from build123d import *

# Parameters (mm, degrees)
SKETCH1_R           = 6
BOSS_EXTRUDE2_DEPTH = 5
SKETCH2_W           = 36
SKETCH2_H           = 12
BOSS_EXTRUDE3_DEPTH = 48
CUT_EXTRUDE1_DEPTH  = 48
SKETCH4_R           = 7.2
CUT_EXTRUDE2_DEPTH  = 48
SKETCH5_R           = 7.2
CUT_EXTRUDE3_DEPTH  = 48


with BuildPart() as part:
    # Sketch1 → Boss-Extrude2 (new body, symmetric)
    with BuildSketch(Plane.XY):
        with BuildLine():
            Line((-48.497409326, 0), (47.502590674, 0))
            Line((47.502590674, 0), (11.523405954, 35.97918472))
            ThreePointArc((11.523405954, 35.97918472), (-0.497409326, 40.95836944), (-12.518224607, 35.97918472))
            Line((-12.518224607, 35.97918472), (-48.497409326, 0))
        make_face()
        with Locations((0, 15)):
            Circle(SKETCH1_R, mode=Mode.SUBTRACT)
    extrude(amount=BOSS_EXTRUDE2_DEPTH, both=True)

    # Sketch2 → Boss-Extrude3 (add, symmetric)
    with BuildSketch(Plane(origin=(0, 0, 0), x_dir=(0, 0, -1), z_dir=(1, 0, 0))):
        with Locations((-13, -6)):
            Rectangle(SKETCH2_W, SKETCH2_H)
    extrude(amount=BOSS_EXTRUDE3_DEPTH, both=True)

    # Sketch3 → Cut-Extrude1 (cut, symmetric)
    with BuildSketch(Plane(origin=(0, 0, 0), x_dir=(1, 0, 0), z_dir=(0, 1, 0))):
        with BuildLine():
            Line((-7, -23), (-7, -31))
            Line((-7, -31), (7, -31))
            Line((7, -31), (7, -23))
            ThreePointArc((7, -23), (4.949747468, -18.050252532), (0, -16))
            ThreePointArc((0, -16), (-4.949747468, -18.050252532), (-7, -23))
        make_face()
    extrude(amount=CUT_EXTRUDE1_DEPTH, both=True, mode=Mode.SUBTRACT)

    # Sketch4 → Cut-Extrude2 (cut, symmetric)
    with BuildSketch(Plane(origin=(0, 0, 0), x_dir=(1, 0, 0), z_dir=(0, 1, 0))):
        with Locations((-36, -18)):
            Circle(SKETCH4_R)
    extrude(amount=CUT_EXTRUDE2_DEPTH, both=True, mode=Mode.SUBTRACT)

    # Sketch5 → Cut-Extrude3 (cut, symmetric)
    with BuildSketch(Plane(origin=(0, 0, 0), x_dir=(1, 0, 0), z_dir=(0, 1, 0))):
        with Locations((36, -18)):
            Circle(SKETCH5_R)
    extrude(amount=CUT_EXTRUDE3_DEPTH, both=True, mode=Mode.SUBTRACT)


solid = part.part
Design review of the part built by this model. Coordinates are the model's own, in mm. A direction names the side the tool comes from. Coordinates: 2 decimals unless noted, no trailing zeros. Loops run counter-clockwise (first coordinate to the right, second up) from the corner with the lowest first, then second, coordinate; pieces in that order, holes last. Notation, with made-up numbers: M -6.5,59.25 L 4.5,59.25 A28 ccw 4.5,97.25 Z; hole C -38,-21 d11. An arc over 180 degrees is marked long. Use one line per item in the form item = value.
(1) Clearance check with flat-ended pins moving along their axes: P1, Ø20.5, axis at x = 4.5, y = 20.5, coming from the +Z side; P2, Ø6.5, axis at y = -6, z = 27, coming from the -X side; P3, Ø6, axis at y = 26.5, z = 4, coming from the +X side. State where each tip first meets the part, or that it passes through.
Return value:
P1 = 5
P2 = -48
P3 = 24
(2) Draft analysis for pull direction Z (two halves, no side actions). For faces 4 (the face through (-41.307, -5.916, 13.134)), 5 (the face through (0, 8, -5)), 6 (the face through (-30.3, 18.2, 0.1)), state which applies: pulls with the +Z half, pulls with the -Z half, needs draft (parallel to the pull), parting line crosses it, or undercut.
Return value:
face_4 = undercut
face_5 = pulls with the -Z half
face_6 = needs draft
(3) Consider section A-A (z = 28). Write out the cut boundary in (x, y), and give its area (3 significant figures).
Return value:
outline = M -48,-12 L -7,-12 L -7,0 L -48,0 Z; M 7,-12 L 48,-12 L 48,0 L 7,0 Z
area = 984 mm2
(4) Consider section C-C (z = 21). Write out the cut boundary in (x, y), and give its area (3 significant figures).
Return value:
outline = M -48,-12 L -42.55,-12 L -42.55,0 L -48,0 Z; M -29.45,-12 L -6.71,-12 L -6.71,0 L -29.45,0 Z; M 6.71,-12 L 29.45,-12 L 29.45,0 L 6.71,0 Z; M 42.55,-12 L 48,-12 L 48,0 L 42.55,0 Z
area = 677 mm2
(5) For line 1 along X through (y, z) = (-5.5, 27); line 2 along Z through (x, y) = (-36, -5.75); line 3 along X through (y, z) = (-4.5, 21), list the stretches that pass through material, from the lowest coordinate up. Write a range as from..to.
Return value:
line_1 = -48..-7, 7..48
line_2 = -5..10.8, 25.2..31
line_3 = -48..-42.55, -29.45..-6.71, 6.71..29.45, 42.55..48
(6) For faces 1 (the face through (-48, -6, 13)), 2 (the face through (-1, 7, 5)), 3 (the face through (-7, -6, 27)), list the 3-axis set-ups (+Z, -Z, +X, -X, +Y, -Y) from which the entire face can be reached by the end or side of a thin tool; tool diameter is ignored.
Return value:
face_1 = +Z, -Z, -X, -Y
face_2 = +Z, +X, -X, +Y
face_3 = +Z, +Y, -Y
(7) Consider section D-D (x = 36). Write out the cut boundary in (y, z).
Return value:
outline = M -12,-5 L 11.5,-5 L 11.5,5 L 0,5 L 0,10.8 L -12,10.8 Z; M -12,25.2 L 0,25.2 L 0,31 L -12,31 Z
(8) Consider section B-B (y = 15). Write out the cut boundary in (x, z), and give its area (3 significant figures).
Return value:
outline = M -33.5,-5 L -6,-5 L -6,5 L -33.5,5 Z; M 6,-5 L 32.5,-5 L 32.5,5 L 6,5 Z
area = 540 mm2
